Could you check a few things on this drawing? It's one solid part, dimensions in mm from its lowest x, y, z. Give positions to 0.01 mm unless a question says otherwise; leave off trailing zeros. Loops run counter-clockwise (first coordinate to the right, second up) from the corner with the lowest first, then second, coordinate; pieces in that order, holes last. Notation, with made-up numbers: (-26.5, -31.75) - (29.5, -31.75) arc R21 cw to (29.5, -19.75) - close; hole circle Ø1 at (75, 20). An arc over 180 degrees is marked (long way). Write each question's results on one line, items separated by ' | '. Start each with the question number.
(1) I need wall thicknesses on line 1 (Y direction, x = 12.7, z = 2.25); line 2 (X direction, y = 6, z = 4.25); line 3 (Y direction, x = 12.75, z = 6) (3 decimals). Which ranges of each line are inside material? Lowest first, please.
(2) Suppose I cut it at B-B (x = 12.7). Please give me the cut outline in (y, z) (3 decimals).
(3) For pin 1 (1.1 mm diameter, centred on x = 4.445, y = 5.842, fed in from -Z), with a flat end and sliding along its axis, tell me the tip position at first contact or that it passes through.
(4) Suppose I cut it at A-A (y = 63.5). Please give me the cut outline in (x, z).
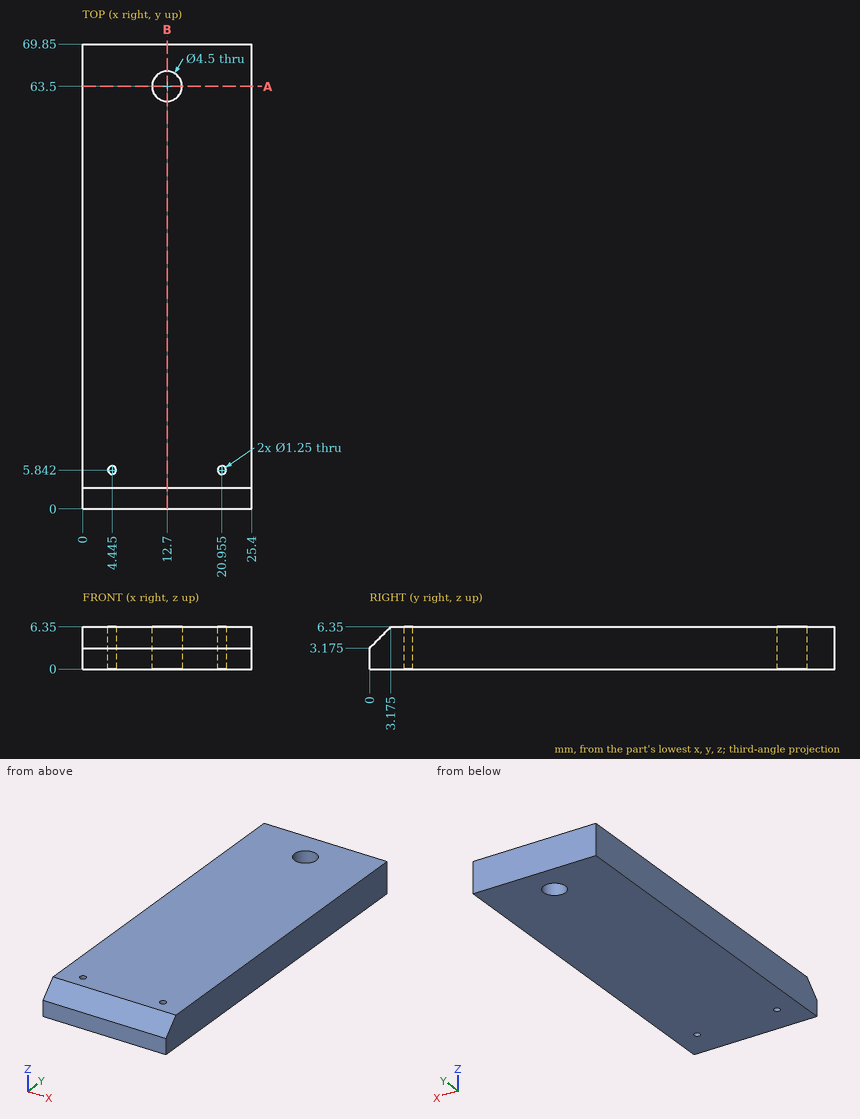
Output values:
1) line 1: 0 to 61.25, 65.75 to 69.85 | line 2: 0 to 3.84, 5.05 to 20.35, 21.56 to 25.4 | line 3: 2.825 to 61.251, 65.749 to 69.85
2) outline: (0, 0) - (61.25, 0) - (61.25, 6.35) - (3.175, 6.35) - (0, 3.175) - close; (65.75, 0) - (69.85, 0) - (69.85, 6.35) - (65.75, 6.35) - close
3) pin 1: through
4) outline: (0, 0) - (10.45, 0) - (10.45, 6.35) - (0, 6.35) - close; (14.95, 0) - (25.4, 0) - (25.4, 6.35) - (14.95, 6.35) - close
